Build history of the part. All positions in model axes, mm. Face numbers are marked on the shaded views. Give positions to 0.01 mm unless a question says otherwise; leave off trailing zeros. Use a Markdown table: item, result. Add a question column.
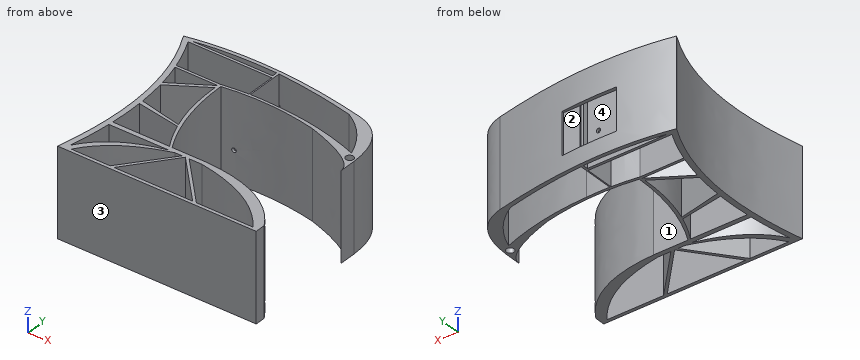
Autodesk Inventor part; units mm, degrees
ref_plane "Work Plane1" through (224.5173, 1793.6598, 410) normal (0, 1, 0) x (-1, 0, 0)
ref_plane "Work Plane2" through (536.3949, 1390.2254, 410) normal (0, -1, 0) x (1, 0, 0)
ref_plane "YZ Plane" through (0, 0, 0) normal (1, 0, 0) x (0, 1, 0)
sketch "Sketch1" plane through (0, 0, 0) normal (0, 0, 1) x (1, 0, 0)
  line L0 (161.1386, 1359.5266) -> (-238.8614, 1359.5266)
  line L1 (161.1386, 1359.5266) -> (-238.8612, 1359.5253)
  line L2 (161.1386, 1359.5266) -> (-238.8613, 1359.5262)
  line L3 (161.1386, 1359.5266) -> (-186.8113, 1142.5066)
  line L4 (248.1161, 771.1351) -> (-152.7891, 857.8121)
  line L5 (-158.5114, 459.5266) -> (400, 459.5266)
  line L6 (-32.9752, 356.2519) -> (400, 459.5266) construction
  spline S0 degree 2 poles (-213.6716, 65.4814) (-32.9752, 356.2519) (400, 459.5266) knots 1.098111 1.098111 1.098111 2 2 2
  line L7 (554.959, 459.5266) -> (223.1733, 30)
  line L8 (554.959, 459.5266) -> (955.815, 30)
  line L9 (400, 1709.5266) -> (-348.1283, 1709.5266)
  line L10 (1559.9999, 1359.5314) -> (1560, 1359.5266)
  line L11 (411.1386, 1410.8176) -> (411.1386, 1509.5266)
  spline S1 degree 2 poles (185.1086, 1363.3695) (609.3989, 1429.0606) (1059.8291, 1334.0674) knots 1.017817 1.017817 1.017817 1.648016 1.648016 1.648016
  line L12 (161.1386, 1383.5266) -> (284.9875, 1404.0635) construction
  spline S2 degree 2 poles (1488.6321, 1252.6922) (1391.0237, 1521.0798) (1159.9182, 1648.2945) knots 1.336028 1.336028 1.336028 1.795606 1.795606 1.795606
  line L13 (1391.0237, 1521.0798) -> (1159.9182, 1648.2945) construction
  line L14 (768.5954, 1734.2188) -> (1159.9182, 1648.2945) construction
  line L15 (1571.1386, 1017.4432) -> (1571.1386, 1177.8289) construction
  line L16 (1571.1386, 1177.8289) -> (1059.8291, 1334.0674) construction
  spline S3 degree 2 poles (1571.1386, 1017.4432) (1571.1386, 1177.8289) (1059.8291, 1334.0674) knots 1 1 1 2 2 2
  line L17 (609.3989, 1429.0606) -> (1059.8291, 1334.0674) construction
  line L18 (1571.1386, 1177.8289) -> (1560, 1593.335) construction
  line L19 (1560, 1593.335) -> (1242.767, 1672.0837) construction
  spline S4 degree 2 poles (1571.1386, 1177.8289) (1560, 1593.335) (1242.767, 1672.0837) knots 1 1 1 2 2 2
  line L20 (1087.8258, 1400.6409) -> (1488.6321, 1252.6922) construction
  spline S5 degree 2 poles (640.5331, 1411.2721) (1087.8258, 1400.6409) (1488.6321, 1252.6922) knots 1.347915 1.347915 1.347915 2 2 2
  line L21 (1488.6321, 1252.6922) -> (1391.0237, 1521.0798) construction
  line L22 (530.6033, 1416.646) -> (640.5331, 1411.2721) construction
  line L23 (640.5331, 1411.2721) -> (1087.8258, 1400.6409) construction
  line L24 (422.363, 1411.9058) -> (422.363, 1757.1534)
  line L25 (411.1386, 1685.5266) -> (-369.8693, 1685.5266)
  line L26 (-295.5796, 1541.4626) -> (-369.8693, 1685.5266) construction
  line L27 (411.1386, 1509.5266) -> (411.1386, 1685.5266)
  line L28 (400, 1709.5266) -> (400, 1758.5718)
  spline S6 degree 2 poles (422.363, 1757.1534) (768.5954, 1734.2188) (1159.9182, 1648.2945) knots 1.466086 1.466086 1.466086 1.822751 1.822751 1.822751
  line L29 (422.363, 1757.1534) -> (768.5954, 1734.2188) construction
  spline S7 degree 2 poles (161.1386, 1383.5266) (284.9875, 1404.0635) (411.1386, 1410.8176) knots 1 1 1 1.184521 1.184521 1.184521
  spline S8 degree 2 poles (422.363, 1411.9058) (530.6033, 1416.646) (640.5331, 1411.2721) knots 1.200863 1.200863 1.200863 1.358931 1.358931 1.358931
  line L30 (284.9875, 1404.0635) -> (411.1386, 1410.8176) construction
  line L31 (422.363, 1411.9058) -> (530.6033, 1416.646) construction
  line L32 (161.1386, 1383.5266) -> (-246.1978, 1383.5266)
  spline S9 degree 2 poles (-246.1978, 1383.5266) (-295.5796, 1541.4626) (-369.8693, 1685.5266) knots 1.776248 1.776248 1.776248 1.982731 1.982731 1.982731
  line L33 (-207.3568, 1254.0684) -> (-238.8614, 1359.5266) construction
  line L34 (-246.1978, 1383.5266) -> (-295.5796, 1541.4626) construction
  line L35 (-30.322, 1016.0709) -> (-60.322, 1016.0709)
  line L36 (-280, 0) -> (-60.322, 1016.0709) construction
  line L37 (-60.322, 1016.0709) -> (-435.5436, 1709.5266) construction
  spline S10 degree 2 poles (-280, 0) (-60.322, 1016.0709) (-435.5436, 1709.5266) knots 1 1 1 2 2 2
  line L38 (1242.767, 1672.0837) -> (287.4624, 1884.9388) construction
  line L39 (287.4624, 1884.9388) -> (-443.9851, 1725.1277) construction
  spline S11 degree 2 poles (1242.767, 1672.0837) (287.4624, 1884.9388) (-443.9851, 1725.1277) knots 1 1 1 2 2 2
  line L40 (-435.5436, 1709.5266) -> (-435.5436, 1718.9513) construction
  line L41 (-435.5436, 1718.9513) -> (-443.9851, 1725.1277) construction
  spline S12 degree 2 poles (-435.5436, 1709.5266) (-435.5436, 1718.9513) (-443.9851, 1725.1277) knots 1 1 1 2 2 2
  line L42 (400, 1758.5718) -> (-26.9296, 1771.5095) construction
  line L43 (-26.9296, 1771.5095) -> (-348.1283, 1709.5266) construction
  spline S13 degree 2 poles (400, 1758.5718) (-26.9296, 1771.5095) (-348.1283, 1709.5266) knots 1 1 1 2 2 2
  line L44 (-213.6716, 65.4814) -> (-32.9752, 356.2519) construction
  line L45 (186.4589, 881.5156) -> (185.1086, 1362.7988) construction
  spline S14 degree 2 poles (397.7918, 502.1083) (186.4589, 881.5156) (185.1086, 1362.7988) knots 1.053519 1.053519 1.053519 2 2 2
  line L46 (185.1086, 1362.7988) -> (185.1086, 1363.3695)
  line L47 (185.1086, 1363.3695) -> (609.3989, 1429.0606) construction
  line L48 (-180.8353, 1108.5501) -> (163.0717, 1326.6666)
  line L49 (160.6844, 1325.1525) -> (159.3113, 1026.732) construction
  spline S15 degree 2 poles (-186.8113, 1142.5066) (-207.3568, 1254.0684) (-238.8614, 1359.5266) knots 1.623647 1.623647 1.623647 1.760611 1.760611 1.760611
  line L50 (-160.3886, 986.7586) -> (-180.8353, 1108.5501) construction
  line L51 (-186.8113, 1142.5066) -> (-207.3568, 1254.0684) construction
  line L52 (256.1307, 748.6567) -> (-150.7068, 816.8479)
  spline S16 degree 2 poles (-152.7891, 857.8121) (-160.3886, 986.7586) (-180.8353, 1108.5501) knots 1.454595 1.454595 1.454595 1.602889 1.602889 1.602889
  line L53 (-144.1812, 664.3923) -> (-150.7068, 816.8479) construction
  line L54 (-152.7891, 857.8121) -> (-160.3886, 986.7586) construction
  spline S17 degree 2 poles (160.6844, 1325.1525) (159.3113, 1026.732) (248.1161, 771.1351) knots 1.033706 1.033706 1.033706 1.621351 1.621351 1.621351
  spline S18 degree 2 poles (256.1307, 748.6567) (303.2321, 619.8647) (373.5724, 502.1083) knots 1.647287 1.647287 1.647287 1.945599 1.945599 1.945599
  line L55 (159.3113, 1026.732) -> (248.1161, 771.1351) construction
  line L56 (256.1307, 748.6567) -> (303.2321, 619.8647) construction
  line L57 (-155.3033, 502.1083) -> (373.5724, 502.1083)
  line L58 (303.2321, 619.8647) -> (373.5724, 502.1083) construction
  spline S19 degree 2 poles (-213.6716, 65.4814) (-174.1396, 269.1604) (-158.5114, 459.5266) knots 1.032347 1.032347 1.032347 1.234626 1.234626 1.234626
  spline S20 degree 2 poles (-155.3033, 502.1083) (-144.1812, 664.3923) (-150.7068, 816.8479) knots 1.257338 1.257338 1.257338 1.431143 1.431143 1.431143
  line L59 (-174.1396, 269.1604) -> (-158.5114, 459.5266) construction
  line L60 (-155.3033, 502.1083) -> (-144.1812, 664.3923) construction
  line L61 (-175.497, 30) -> (3.3356, 317.7714) construction
  line L62 (3.3356, 317.7714) -> (456.7489, 459.5266) construction
  spline S21 degree 2 poles (-175.497, 30) (3.3356, 317.7714) (456.7489, 459.5266) knots 1 1 1 2 2 2
  line L63 (397.7918, 502.1083) -> (718.4486, 502.1083)
  line L64 (1571.1386, 95.1334) -> (1336.4814, 481.3927) construction
  line L65 (1336.4814, 481.3927) -> (718.4486, 502.1083) construction
  spline S22 degree 2 poles (1571.1386, 95.1334) (1336.4814, 481.3927) (718.4486, 502.1083) knots 1 1 1 2 2 2
  line L66 (397.7918, 502.1083) -> (186.4589, 881.5156) construction
  line L67 (1516.7362, 30) -> (1275.4709, 372.4307) construction
  line L68 (1275.4709, 372.4307) -> (709.9179, 459.5266) construction
  spline S23 degree 2 poles (1516.7362, 30) (1275.4709, 372.4307) (709.9179, 459.5266) knots 1 1 1 2 2 2
  line L69 (-213.6716, 65.4814) -> (-174.1396, 269.1604) construction
  line L70 (1571.1386, 0) -> (1571.1386, 95.1334)
  line L71 (1571.1386, 1017.4432) -> (1571.1386, 1177.8289)
  line L72 (186.4589, 30) -> (524.6326, 459.5266)
  line L73 (589.667, 459.5266) -> (990.523, 30)
  line L74 (709.9179, 459.5266) -> (589.667, 459.5266)
  line L75 (524.6326, 459.5266) -> (456.7489, 459.5266)
  line L76 (-175.497, 30) -> (186.4589, 30)
  line L77 (223.1733, 30) -> (955.815, 30)
  line L78 (990.523, 30) -> (1516.7362, 30)
  circle A0 centre (1516.7362, 1194.4524) radius 36
  line L79 (-280, 0) -> (1571.1386, 0)
  point P0 (390.9108, 1423.4749)
  point P1 (271.3597, 1843.399)
  point P2 (-16.2977, 999.8731)
  point P3 (-67.3038, 785.2568)
  point P4 (158.4265, 834.4446)
  point P5 (-99.7467, 625.5419)
  point P6 (-135.0742, 451.6261)
  dimension "d13" = 400
  dimension "d25" = 30
  dimension "d27" = 72
extrude "Extrusion1" add sketch "Sketch1" along normal blind 820
ref_plane "Work Plane1" through (224.5173, 1793.6598, 410) normal (0, 1, 0) x (-1, 0, 0)
sketch "Sketch2" plane through (224.5173, 1793.6598, 410) normal (0, 1, 0) x (-1, 0, 0)
  line L0 (159.536, -258.0302) -> (-360.464, -258.0302)
  line L1 (-360.464, -258.0302) -> (-360.464, 133.9698)
  line L2 (-360.464, 133.9698) -> (159.536, 133.9698)
  line L3 (159.536, 133.9698) -> (159.536, -258.0302)
  point P0 (224.5173, -410)
  dimension "d30" = 520
  dimension "d31" = 392
extrude "Extrusion2" cut sketch "Sketch2" against normal blind 37.25
ref_plane "Work Plane2" through (536.3949, 1390.2254, 410) normal (0, -1, 0) x (1, 0, 0)
sketch "Sketch3" plane through (536.3949, 1390.2254, 410) normal (0, -1, 0) x (1, 0, 0)
  circle A0 centre (-239.5375, -116.5899) radius 20
  point P0 (-536.3949, -410)
  dimension "d34" = 40
extrude "Extrusion3" cut sketch "Sketch3" along normal mid plane 874.75
properties part number "silla"
(1) Pin check, flat tip, straight feed: pin 1 Ø11 at (x, z) = (415.5, 259.5) entering from +Y. Stop position of the tip, or through.
(2) Mould opens along Y. For the marked faces 1, 2, 3 and 4 say: released by +Y, released by -Y, zero draft, split by the parting line, or undercut.
(3) Wall check: probe 1 along Y at (x, z) = (622, 415); probe 2 along X at (y, z) = (107, 249); probe 3 along Y at (x, z) = (1445, 660). Give the ranges that are in metal, low to high.
(4) Band-saw the part on A-A on x = 129. State how many separate pieces and enclosed holes the cut face has, plus the area to 3 significant figures.
Response:
| question | item | result |
|---|---|---|
| 1 | pin 1 | stops at y = 1756.41 |
| 2 | face 1 | undercut |
| 2 | face 2 | released by +Y |
| 2 | face 3 | released by -Y |
| 2 | face 4 | undercut |
| 3 | probe 1 | y = 0 to 30, 387.69 to 424.88, 459.53 to 502.11, 1388.68 to 1412.11, 1739.12 to 1773.45 |
| 3 | probe 2 | x = -258.35 to -205.84, -185.9 to -120.62, 247.08 to 282.65, 883.95 to 918.66, 1455.51 to 1563.78 |
| 3 | probe 3 | y = 0 to 30, 118.54 to 251.52, 1175.74 to 1268.34, 1352.95 to 1558 |
| 4 | separate pieces | 9 |
| 4 | enclosed holes | 0 |
| 4 | area | 202,000 mm² |
